For this review, use the dimensioned drawing (mm, ordinates from the lowest corner) and the shaded views. Give positions to 0.01 mm unless a question says otherwise; leave off trailing zeros. Loops run counter-clockwise (first coordinate to the right, second up) from the corner with the lowest first, then second, coordinate; pieces in that order, holes last. Notation, with made-up numbers: (68.25, 71.5) -> (102.25, 71.5) arc R29 cw to (102.25, 91.5) -> close; hole circle Ø9 at (73.25, 34.5). An arc over 180 degrees is marked (long way). Write each question's results on one line, items separated by ' | '. Start each with the question number.
Q1. We need section C-C (x = 20). Write out the cut boundary in (y, z) (1 decimal), plus the area to 3 significant figures.
Q2. We need section D-D (x = 6.5). Write out the cut boundary in (y, z), plus the area to 3 significant figures.
Q3. We need section A-A (z = 1.4). Write out the cut boundary in (x, y) (1 decimal).
Q4. Wall thickness on L1, parallel to Y at x = 34, z = 4.75; L2, parallel to Y at x = 24, z = 4; L3, parallel to X at y = 11.5, z = 3.6 (1 decimal): over which ranges is each line inside the solid? List them lowest first. Write a range as [from, to].
Q5. Insertion check: pin 1 Ø2 at (x, z) = (30, 1.5) entering from -Y; pin 2 Ø3 at (y, z) = (10.5, 1) entering from +X; pin 3 Ø1.5 at (x, z) = (6.5, 4) entering from +Y (1 decimal); pin 4 Ø12 at (x, y) = (11, 36.5) entering from -Z. Each pin has a flat end and moves straight along its axis. Give the tip position at first contact, or say it passes through.
Q6. We need section B-B (y = 34). Write out the cut boundary in (x, z).
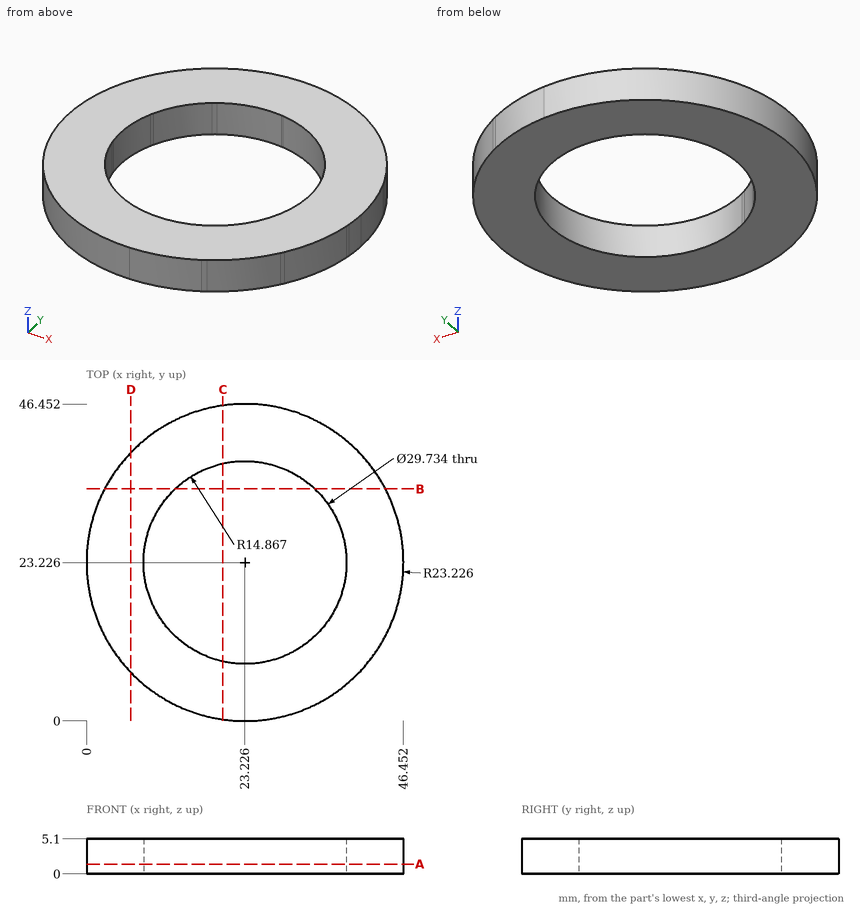
Output:
1) outline: (0.2, 0) -> (8.7, 0) -> (8.7, 5.1) -> (0.2, 5.1) -> close; (37.7, 0) -> (46.2, 0) -> (46.2, 5.1) -> (37.7, 5.1) -> close | area: 86.6 mm2
2) outline: (7.11, 0) -> (39.34, 0) -> (39.34, 5.1) -> (7.11, 5.1) -> close | area: 164 mm2
3) outline: circle Ø46.5 at (23.2, 23.2); hole circle Ø29.7 at (23.2, 23.2)
4) L1: [2.65, 12.98], [33.47, 43.8] | L2: [0.01, 8.38], [38.07, 46.44] | L3: [3.2, 14.1], [32.4, 43.3]
5) pin 1: y = 0.73 | pin 2: x = 43.56 | pin 3: y = 40.1 | pin 4: z = 0
6) outline: (2.65, 0) -> (12.98, 0) -> (12.98, 5.1) -> (2.65, 5.1) -> close; (33.47, 0) -> (43.8, 0) -> (43.8, 5.1) -> (33.47, 5.1) -> close
